Part model, mm, in its own coordinate system. A direction names the side the tool comes from. Coordinates: 2 decimals unless noted, no trailing zeros. Loops run counter-clockwise (first coordinate to the right, second up) from the corner with the lowest first, then second, coordinate; pieces in that order, holes last. Notation, with made-up numbers: M 31.25,81 L 37.25,81 A18 cw 37.25,100 Z; hole C 77.5,-39.75 d5. An arc over 180 degrees is marked long. Use a Markdown table: item, result. Add a question column.
1) Wall check: probe 1 along Y at (x, z) = (6.5, 0.4); probe 2 along Y at (x, z) = (-3.5, 0.6); probe 3 along X at (y, z) = (-0.5, 0.1). Give the ranges that are in metal, low to high. Write a range as from..to.
2) Band-saw the part on B-B (z = 0.2). List the corners of the cut face in (x, y).
3) Tool access for faces 1 (the flat face through (4, 4, 1)), 2 (the flat face through (-5, 4, 1)), 3 (the flat face through (2.5, -4.5, 0.7)): list every direction of +Z, -Z, +X, -X, +Y, -Y with a clear straight run to the whole face (end or side of a thin tool).
4) Pull direction Y, two halves, no side cores. Call faces 4 (the cylindrical face through (5.253, -0.517, 0.739)), 5 (the flat face through (2.5, 4.5, 0.7)), 6 (the cylindrical face through (10.5, 0.1, 0.7)): released by +Y, released by -Y, zero draft, split by the parting line, or undercut.
5) Band-saw the part on D-D (y = 1). List the corners of the cut face in (x, z), plus the area to 3 significant figures.
6) Band-saw the part on C-C (x = 4.5). List the corners of the cut face in (y, z).
7) Band-saw the part on A-A (y = 0). List the corners of the cut face in (x, z).
8) Pin check, flat tips, straight feed: pin 1 Ø0.5 at (y, z) = (4.5, 0.5) entering from +X; pin 2 Ø0.5 at (y, z) = (-4.5, 1) entering from -X; pin 3 Ø5 at (x, y) = (8, 0) entering from -Z. Stop position of each tip, or through.
from build123d import *

# Parameters (mm, degrees)
SKETCH_1_W           = 8
SKETCH_1_H           = 8
SKETCH_1_W_2         = 5
SKETCH_1_H_2         = 10
EXTRUDE_709_DEPTH    = 1.5
HOLE_WIZARD_M2_5_1_D = 2.7
FILLET_1_RADIUS      = 4
FILLET_1_LENGTH      = 1.5
FILLET_2_RADIUS      = 4
FILLET_2_LENGTH      = 1.5
FILLET_START         = -1.4
FILLET_3_DEPTH       = 2.8


with BuildPart() as part:
    # 草图1 → Extrude 709 (new body)
    with BuildSketch(Plane.XY):
        with Locations((6.5, 0)):
            Rectangle(SKETCH_1_W, SKETCH_1_H)
        Rectangle(SKETCH_1_W_2, SKETCH_1_H_2)
        with Locations((-6.5, 0)):
            Rectangle(SKETCH_1_W, SKETCH_1_H)
    extrude(amount=EXTRUDE_709_DEPTH)

    # M2.5 间隙孔1 (through all)
    with Locations(Plane.XY.offset(1.5)):
        with Locations((6.5, 0)):
            hole_wizard_m2_5_1 = Hole(HOLE_WIZARD_M2_5_1_D / 2)

    # 镜向2: M2.5 间隙孔1 across plane
    add(hole_wizard_m2_5_1.mirror(Plane(origin=(0, 0, 0), x_dir=(0, 0, 1), z_dir=(1, 0, 0))), mode=Mode.SUBTRACT)

    # 圆角1: full round fillet: the end face becomes a half cylinder, R = half its width
    fillet_1_face = Plane((10.5, 0, 0.75), x_dir=(0, 0, -1), z_dir=(1, 0, 0))  # on the end face: x along it, z out of the body
    fillet_1_slab = fillet_1_face.offset(-FILLET_1_RADIUS / 2) * Box(FILLET_1_LENGTH, 2 * FILLET_1_RADIUS, FILLET_1_RADIUS, mode=Mode.PRIVATE)  # the body's end, R deep
    fillet_1_round = Plane((6.5, 0, 0.75), x_dir=(1, 0, 0), z_dir=(0, 0, -1)) * Cylinder(FILLET_1_RADIUS, FILLET_1_LENGTH, mode=Mode.PRIVATE)  # its axis R under the face
    add(fillet_1_slab - fillet_1_round, mode=Mode.SUBTRACT)

    # 圆角2: full round fillet: the end face becomes a half cylinder, R = half its width
    fillet_2_face = Plane((-10.5, 0, 0.75), x_dir=(0, 0, 1), z_dir=(-1, 0, 0))  # on the end face: x along it, z out of the body
    fillet_2_slab = fillet_2_face.offset(-FILLET_2_RADIUS / 2) * Box(FILLET_2_LENGTH, 2 * FILLET_2_RADIUS, FILLET_2_RADIUS, mode=Mode.PRIVATE)  # the body's end, R deep
    fillet_2_round = Plane((-6.5, 0, 0.75), x_dir=(-1, 0, 0), z_dir=(0, 0, 1)) * Cylinder(FILLET_2_RADIUS, FILLET_2_LENGTH, mode=Mode.PRIVATE)  # its axis R under the face
    add(fillet_2_slab - fillet_2_round, mode=Mode.SUBTRACT)

    # 圆角3: read off the stored shape, not the designer's step
    # 圆角3 outline → 圆角3 (cut)
    with BuildSketch(Plane.YZ.offset(FILLET_START)):
        with BuildLine():
            Line((5, 0), (5, 0.5))
            ThreePointArc((5, 0.5), (4.853553391, 0.146446609), (4.5, 0))
            Line((4.5, 0), (5, 0))
        make_face()
        with BuildLine():
            Line((-5, 0), (-4.5, 0))
            ThreePointArc((-4.5, 0), (-4.853553391, 0.146446609), (-5, 0.5))
            Line((-5, 0.5), (-5, 0))
        make_face()
    extrude(amount=FILLET_3_DEPTH, mode=Mode.SUBTRACT)


solid = part.part
Entries:
| question | item | result |
|---|---|---|
| 1 | probe 1 | -4..-1.35, 1.35..4 |
| 1 | probe 2 | -4..4 |
| 1 | probe 3 | -10.47..-7.75, -5.25..5.25, 7.75..10.47 |
| 2 | outline | M -6.5,-4 L -2.5,-4 L -2.5,-5 L -1.4,-5 L -1.4,-4.9 L 1.4,-4.9 L 1.4,-5 L 2.5,-5 L 2.5,-4 L 6.5,-4 A4 ccw 6.5,4 L 2.5,4 L 2.5,5 L 1.4,5 L 1.4,4.9 L -1.4,4.9 L -1.4,5 L -2.5,5 L -2.5,4 L -6.5,4 A4 ccw Z; hole C -6.5,0 d2.7; hole C 6.5,0 d2.7 |
| 3 | face 1 | +Z, -Z, +X, +Y |
| 3 | face 2 | +Z, -Z, -X, +Y |
| 3 | face 3 | +Z, -Z, +X, -Y |
| 4 | face 4 | undercut |
| 4 | face 5 | zero draft |
| 4 | face 6 | split by the parting line |
| 5 | outline | M -10.37,0 L -7.41,0 L -7.41,1.5 L -10.37,1.5 Z; M -5.59,0 L 5.59,0 L 5.59,1.5 L -5.59,1.5 Z; M 7.41,0 L 10.37,0 L 10.37,1.5 L 7.41,1.5 Z |
| 5 | area | 25.7 mm2 |
| 6 | outline | M -4,0 L 4,0 L 4,1.5 L -4,1.5 Z |
| 7 | outline | M -10.5,0 L -7.85,0 L -7.85,1.5 L -10.5,1.5 Z; M -5.15,0 L 5.15,0 L 5.15,1.5 L -5.15,1.5 Z; M 7.85,0 L 10.5,0 L 10.5,1.5 L 7.85,1.5 Z |
| 8 | pin 1 | x = 2.5 |
| 8 | pin 2 | x = -2.5 |
| 8 | pin 3 | z = 0 |
